Could you check a few things on this model? Use its own coordinates, in mm. A direction names the side the tool comes from. Round coordinates to 2 decimals unless told otherwise and drop trailing zeros. Loops run counter-clockwise (first coordinate to the right, second up) from the corner with the lowest first, then second, coordinate; pieces in that order, holes last. Notation, with made-up numbers: M -36.5,-7.75 L 15.5,-7.75 A12 cw 15.5,2.25 Z; hole C -7.5,85 d1. An arc over 180 degrees is marked long. Answer in a Markdown table with one row per item.
```python
from build123d import *

# Parameters (mm, degrees)
SKETCH_4_W          = 26.5
SKETCH_4_H          = 26.5
SKETCH_4_W_2        = 20.5
SKETCH_4_H_2        = 20.5
EXTRUDE_1_DEPTH     = 50
EXTRUDE_2_DEPTH     = 50
EXTRUDE_3_DEPTH     = 17.5
SKETCH_4_2_W        = 20.5
SKETCH_4_2_H        = 20.5
CUT_EXTRUDE_1_DEPTH = 82.971372719
CUT_EXTRUDE_2_DEPTH = 82.971372719
CUT_EXTRUDE_3_REACH = 90.259
SKETCH_7_R          = 1.6
SKETCH_9_R          = 1.6
CUT_EXTRUDE_4_DEPTH = 76.350501248


with BuildPart() as part:
    # 草图4 → 凸台-拉伸1 (new body)
    with BuildSketch(Plane(origin=(0, 0, 0), x_dir=(1, 0, 0), z_dir=(0, 1, 0))):
        Rectangle(SKETCH_4_W, SKETCH_4_H)
        Rectangle(SKETCH_4_W_2, SKETCH_4_H_2, mode=Mode.SUBTRACT)
    extrude(amount=-EXTRUDE_1_DEPTH)

    # 草图5 → 凸台-拉伸2 (add)
    with BuildSketch(Plane(origin=(0, 0, 0), x_dir=(0.7254762501100117, 0.21764287503300356, -0.6529286250990104), z_dir=(0.6882472016116853, -0.22941573387056186, 0.6882472016116854))):
        Polygon((-9.951712437, 15.877292577), (15.877292577, 9.951712437), (9.951712437, -15.877292577), (-15.877292577, -9.951712437), align=None)
        Polygon((-7.698494526, 12.28243388), (12.28243388, 7.698494526), (7.698494526, -12.28243388), (-12.28243388, -7.698494526), align=None, mode=Mode.SUBTRACT)
    extrude(amount=EXTRUDE_2_DEPTH)

    # 草图6 → 凸台-拉伸3 (add, symmetric)
    with BuildSketch(Plane(origin=(0, 0, 0), x_dir=(1, 0, 0), z_dir=(0, 1, 0))):
        Polygon((-13.25, 13.25), (-13.25, -21.75), (3.011670299, -21.75), (21.75, -3.011670299), (21.75, 13.25), align=None)
    extrude(amount=EXTRUDE_3_DEPTH, both=True)

    # 草图4<2> → 切除-拉伸1 (cut, through all)
    with BuildSketch(Plane(origin=(0, 0, 0), x_dir=(1, 0, 0), z_dir=(0, 1, 0))):
        Rectangle(SKETCH_4_2_W, SKETCH_4_2_H)
    extrude(amount=-CUT_EXTRUDE_1_DEPTH, mode=Mode.SUBTRACT)

    # 草图5<2> → 切除-拉伸2 (cut, through all)
    with BuildSketch(Plane(origin=(0, 0, 0), x_dir=(0.7254762501100117, 0.21764287503300356, -0.6529286250990104), z_dir=(0.6882472016116853, -0.22941573387056186, 0.6882472016116854))):
        Polygon((12.28243388, 7.698494526), (7.698494526, -12.28243388), (-12.28243388, -7.698494526), (-7.698494526, 12.28243388), align=None)
    extrude(amount=CUT_EXTRUDE_2_DEPTH, mode=Mode.SUBTRACT)

    # 切除-拉伸3: up to this face of the body (flat: up to its plane)
    cut_extrude_3_end = Plane(part.part.faces().sort_by_distance((22.026190668, -20.955144479, 22.026190668))[0])
    # 草图7 → 切除-拉伸3 (cut, up to the picked face)
    with BuildSketch(Plane(origin=(2.14943383, 12.89660298, 2.14943383), x_dir=(0.9867543820659302, -0.16001422411879954, -0.02666903735313327), z_dir=(0.16222142113076257, 0.9733285267845753, 0.16222142113076257)), mode=Mode.PRIVATE) as cut_extrude_3_sk1:
        with Locations(Location((31.386862461, -32.246935744, 0), (0, 0, 270))):
            Circle(SKETCH_7_R)
    cut_extrude_3_tool1 = split(extrude(cut_extrude_3_sk1.sketch, amount=-CUT_EXTRUDE_3_REACH, mode=Mode.PRIVATE), bisect_by=cut_extrude_3_end, keep=Keep.BOTH, mode=Mode.PRIVATE)
    # 草图7 → 切除-拉伸3 (cut, up to the picked face)
    with BuildSketch(Plane(origin=(2.14943383, 12.89660298, 2.14943383), x_dir=(0.9867543820659302, -0.16001422411879954, -0.02666903735313327), z_dir=(0.16222142113076257, 0.9733285267845753, 0.16222142113076257)), mode=Mode.PRIVATE) as cut_extrude_3_sk2:
        with Locations(Location((20.924574974, -21.497957163, 0), (0, 0, 270))):
            Circle(SKETCH_7_R)
    cut_extrude_3_tool2 = split(extrude(cut_extrude_3_sk2.sketch, amount=-CUT_EXTRUDE_3_REACH, mode=Mode.PRIVATE), bisect_by=cut_extrude_3_end, keep=Keep.BOTH, mode=Mode.PRIVATE)
    add(cut_extrude_3_tool1.solids().sort_by(Axis((33.120558, 2.572895, 33.120558), (-0.16222142113076257, -0.9733285267845753, -0.16222142113076257)))[0], mode=Mode.SUBTRACT)
    add(cut_extrude_3_tool2.solids().sort_by(Axis((22.79685, 6.014131, 22.79685), (-0.16222142113076257, -0.9733285267845753, -0.16222142113076257)))[0], mode=Mode.SUBTRACT)

    # 草图9 → 切除-拉伸4 (cut, through all)
    with BuildSketch(Plane(origin=(13.25, 0, 0), x_dir=(0, 0, -1), z_dir=(1, 0, 0))):
        with Locations((0, -42.5)):
            Circle(SKETCH_9_R)
        with Locations((0, -22.5)):
            Circle(SKETCH_9_R)
    extrude(amount=-CUT_EXTRUDE_4_DEPTH, mode=Mode.SUBTRACT)


solid = part.part
```
1) I want a section at A-A, the plane y = -42.5. Please give me the cut outline in (x, z).
Computed:
| item | result |
|---|---|
| outline | M -13.25,-13.25 L 13.25,-13.25 L 13.25,-1.6 L 10.25,-1.6 L 10.25,-10.25 L -10.25,-10.25 L -10.25,-1.6 L -13.25,-1.6 Z; M -13.25,1.6 L -10.25,1.6 L -10.25,10.25 L 10.25,10.25 L 10.25,1.6 L 13.25,1.6 L 13.25,13.25 L -13.25,13.25 Z |
2) Will these pins go through, and if not, where does the flat tip stop? P1, Ø2, axis at x = 27, y = 9, coming from the -Z side; P2, Ø4, axis at x = -5.5, z = 18, coming from the -Y side; P3, Ø6, axis at y = -36, z = -6, coming from the +X side; P4, Ø13, axis at y = 4, z = -6.5, coming from the +X side.
Computed:
| item | result |
|---|---|
| P1 | passes through |
| P2 | stops at y = -17.5 |
| P3 | stops at x = 13.25 |
| P4 | stops at x = 21.75 |
3) I need wall thicknesses on line 1 (Y direction, x = -12.4, z = 0); line 2 (Y direction, x = 12.5, z = 0); line 3 (X direction, y = -45.5, z = -7). Which ranges of each line are inside material? Lowest first, please.
Computed:
| item | result |
|---|---|
| line 1 | y = -50 to -44.1, -40.9 to -24.1, -20.9 to 17.5 |
| line 2 | y = -50 to -44.1, -40.9 to -24.1, -20.9 to -12.61, 8.45 to 17.5 |
| line 3 | x = -13.25 to -10.25, 10.25 to 13.25 |
4) I want a section at B-B, the plane x = 15. Please give me the cut outline in (y, z).
Computed:
| item | result |
|---|---|
| outline | M -21.74,33.74 L -17.5,8.32 L -17.5,-13.25 L 17.5,-13.25 L 17.5,9.76 L 9.49,9.76 L 5.49,33.74 Z; hole M -17.95,29.5 L -13.11,0.5 L 7.95,0.5 L 3.11,29.5 Z |
5) Which directions (+Z, -Z, +X, -X, +Y, -Y) give clear straight access to the entire face, cutting with the end or side of a thin tool? Please do faces 5 (the face through (-10.25, -25, 0)), 6 (the face through (12.25, 13.55, 12.51)), 7 (the face through (-5, 0, 21.75)), 8 (the face through (24.236, -5.515, 9.741)), 9 (the face through (-4, -17.5, 17)).
Computed:
| item | result |
|---|---|
| face 5 | -Y |
| face 6 | +Z, +X, +Y |
| face 7 | +Z, -X, +Y, -Y |
| face 8 | none |
| face 9 | -X, -Y |
6) If we mould it in two halves opening along Y, with no side actions, what happens to faces 1 (the face through (12, -50, 0)), 2 (the face through (24.171, 5.512, 24.433)), 3 (the face through (27.668, -21.634, 29.835)), 4 (the face through (0, -30, 10.25))? For each: released by +Y, released by -Y, zero draft, split by the parting line, or undercut.
Computed:
| item | result |
|---|---|
| face 1 | released by -Y |
| face 2 | released by +Y |
| face 3 | undercut |
| face 4 | zero draft |
7) I want a section at C-C, the plane z = 0. State how many separate pieces and enclosed holes the cut face has, plus the area to 3 significant figures.
Computed:
| item | result |
|---|---|
| separate pieces | 5 |
| enclosed holes | 0 |
| area | 852 mm² |
8) I want a section at D-D, the plane z = 12. Please give me the cut outline in (x, y).
Computed:
| item | result |
|---|---|
| outline | M -13.25,-50 L 13.25,-50 L 13.25,-17.82 L 30.74,-20.74 L 30.74,6.49 L 12.76,9.49 L 12.76,17.5 L -13.25,17.5 Z; hole M -2.5,-12.11 L 26.5,-16.95 L 26.5,4.11 L -2.5,8.95 Z |
